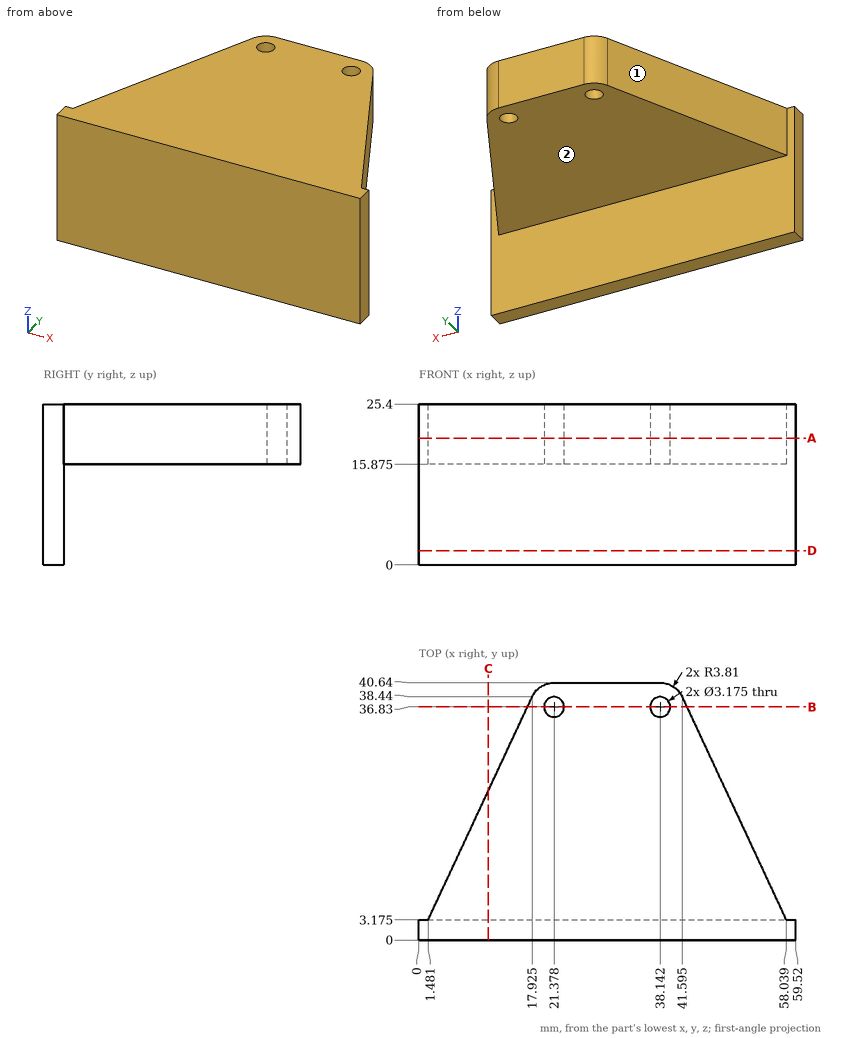
Verification items for this drawing (mm, ordinates from the low corner). A direction names the side the tool comes from. Coordinates: 2 decimals unless noted, no trailing zeros. Order: outer loops, then holes, each group sorted by start corner. A loop starts at its lowest first (then second) coordinate and runs counter-clockwise, first axis right, second up. Notation, with made-up numbers: M 11.5,-17.75 L 18.5,-17.75 A17 ccw 18.5,-3.75 Z; hole C 48,-30 d11. An arc over 180 degrees is marked long. One line per item, written item: value. Start each with the question number.
Item 1: Access from +Z, -Z, +X, -X, +Y, -Y to the whole of each face (thin tool, end or side, straight path). Record for the marked faces 1 and 2.
Item 2: Thickness scan on probe 1 along Y at (x, z) = (31, 2) (1 decimal); probe 2 along Z at (x, y) = (18, 13) (1 decimal); probe 3 along Y at (x, z) = (37.5, 24). Record the ranges inside material, lowest first.
Item 3: Depth check by flat-ended pin: P1, Ø3, axis at x = 21.38, y = 36.83, coming from the +Z side; P2, Ø8, axis at x = 10.5, y = 31.5, coming from the -Z side (3 decimals); P3, Ø3, axis at y = 33.5, z = 17, coming from the -X side; P4, Ø8, axis at x = 37, z = 3, coming from the +Y side (3 decimals). Enter the tip coordinate at first touch or a pass-through.
Item 4: Sectioned sample at C-C on x = 11. Record the cut outline in (y, z) (1 decimal).
Item 5: Sectioned sample at B-B on y = 36.83. Record the cut outline in (x, z) (1 decimal), then the cut area to 3 significant figures.
Item 6: Sectioned sample at A-A on z = 20. Record the cut outline in (x, y) (1 decimal), then the cut area to 3 significant figures.
Item 7: Sectioned sample at D-D on z = 2.25. Record the cut outline in (x, y) (1 decimal).
Calculated:
1. face 1: +Z, -Z, -X, +Y
1. face 2: -Z, +X, -X, +Y
2. probe 1: 0 to 3.2
2. probe 2: 15.9 to 25.4
2. probe 3: 0 to 35.38, 38.28 to 40.64
3. P1: through
3. P2: z = 15.875
3. P3: x = 14.92
3. P4: y = 3.175
4. outline: M 0,0 L 3.2,0 L 3.2,15.9 L 23.6,15.9 L 23.6,25.4 L 0,25.4 Z
5. outline: M 17.2,15.9 L 19.8,15.9 L 19.8,25.4 L 17.2,25.4 Z; M 23,15.9 L 36.6,15.9 L 36.6,25.4 L 23,25.4 Z; M 39.7,15.9 L 42.3,15.9 L 42.3,25.4 L 39.7,25.4 Z
5. area: 179 mm^2
6. outline: M 0,0 L 59.5,0 L 59.5,3.2 L 58,3.2 L 41.6,38.4 A3.8 ccw 38.1,40.6 L 21.4,40.6 A3.8 ccw 17.9,38.4 L 1.5,3.2 L 0,3.2 Z; hole C 21.4,36.8 d3.2; hole C 38.1,36.8 d3.2
6. area: 1,640 mm^2
7. outline: M 0,0 L 59.5,0 L 59.5,3.2 L 0,3.2 Z
